Autodesk Inventor part; units mm, degrees
ref_plane "YZ Plane" through (0, 0, 0) normal (1, 0, 0) x (0, 1, 0)
ref_plane "XZ Plane" through (0, 0, 0) normal (0, 1, 0) x (-1, 0, 0)
ref_plane "XY Plane" through (0, 0, 0) normal (0, 0, 1) x (1, 0, 0)
sketch "Sketch1" plane through (0, 0, 0) normal (0, 0, 1) x (1, 0, 0)
  line L0 (-6.55, 3.425) -> (6.55, 3.425)
  line L1 (6.55, 3.425) -> (6.55, -3.425)
  line L2 (6.55, -3.425) -> (-6.55, -3.425)
  line L3 (-6.55, -3.425) -> (-6.55, 3.425)
  point P0 (0, 0)
  dimension "d0" = 13.1
  dimension "d1" = 6.85
  dimension "d2" = 3.425
  dimension "d3" = 6.55
extrude "Extrusion1" add sketch "Sketch1" along normal blind 14.15
sketch "Sketch2" plane through (0, 0, 14.15) normal (0, 0, 1) x (1, 0, 0)
  line L0 (-6, 2.5343) -> (6, 2.5343)
  line L1 (6, 2.5343) -> (6, -2.425)
  line L2 (6, -2.425) -> (-6, -2.425)
  line L3 (-6, -2.425) -> (-6, 2.5343)
  line L4 (-6.55, -3.425) -> (6.55, -3.425)
  line L5 (6.55, 3.425) -> (-6.55, 3.425)
  point P0 (0, 0)
  dimension "d7" = 12
  dimension "d8" = 6
  dimension "d9" = 1
extrude "Extrusion2" cut sketch "Sketch2" against normal blind 10
sketch "Sketch3" plane through (0, 0, 4.15) normal (0, 0, 1) x (1, 0, 0)
  line L0 (-4.7039, 1.4576) -> (5.0017, 1.4576)
  line L1 (5.0017, 1.4576) -> (5.0017, 0.3455)
  line L2 (5.0017, 0.3455) -> (-4.7039, 0.3455)
  line L3 (-4.7039, 0.3455) -> (-4.7039, 1.4576)
  point P0 (0, 0)
extrude "Extrusion3" add sketch "Sketch3" along normal blind 8
sketch "Sketch4" plane through (6.55, -3.425, 0) normal (1, 0, 0) x (0, 0, -1)
  line L0 (-4.85, 2.838) -> (-2.85, 2.838)
  line L1 (-2.85, 2.838) -> (-2.85, -3.2)
  line L2 (-2.85, -3.2) -> (-4.85, -3.2)
  line L3 (-4.85, -3.2) -> (-4.85, 2.838)
  line L4 (-14.15, 0) -> (-14.15, 6.85)
  arc A0 (-4.85, -2.2) -> (-2.85, -2.2) centre (-3.85, -2.2) ccw
  point P0 (0, 3.425)
  dimension "d17" = 2
  dimension "d18" = 9.3
  dimension "d21" = 3.2
extrude "Extrusion4" add sketch "Sketch4" against normal blind 0.5 contours L0 L1 A0 L3
sketch "Sketch5" plane through (-6.55, -3.425, 0) normal (0, -1, 0) x (1, 0, 0)
  line L0 (13.8244, -1.52) -> (1.8735, -1.52) construction
  line L1 (13.8244, 1.1) -> (1.8735, 1.1) construction
  line L2 (13.1, 4.85) -> (12.6, 4.85)
  circle A0 centre (5.55, 1.1) radius 0.4
  circle A1 centre (7.55, 1.1) radius 0.4
  circle A2 centre (3.05, 1.1) radius 0.4
  circle A3 centre (10.05, 1.1) radius 0.4
  point P0 (6.55, 0)
  dimension "d25" = 2.62
  dimension "d26" = 3.75
  dimension "d29" = 2
  dimension "d30" = 1
  dimension "d31" = 2.5
  dimension "d34" = 2.5
  dimension "d35" = 0.8
  dimension "d36" = 0.8
  dimension "d40" = 0.8
  dimension "d42" = 0.8
extrude "Extrusion5" add sketch "Sketch5" along normal blind 3.2
mirror "Mirror1" about plane through (0, 0, 0) normal (1, 0, 0) of "Extrusion4"
properties part number "USBA_CNC"
Source: CAD feature listing. Evaluate the final solid. Frame: model axes, mm. A direction names the side the tool comes from. Coordinates: 2 decimals unless noted, no trailing zeros. Loops run counter-clockwise (first coordinate to the right, second up) from the corner with the lowest first, then second, coordinate; pieces in that order, holes last. Notation, with made-up numbers: M -18,-28 L -9,-28 A13 ccw -9,-24 Z; hole C 87.5,-23 d8. An arc over 180 degrees is marked long. Put each result on its own line as item: value. Start each with the question number.
1) Contact query for flat-ended pins moving along their axis: pin 1 Ø3 at (x, z) = (3, 11.5) entering from -Y (3 decimals); pin 2 Ø1.5 at (x, y) = (-2, 0.5) entering from +Z. Output: stop coordinate, or through.
2) Pull-direction query (Y, two-part tool) for faces 1 (the face through (-4.704, 1, 8)), 2 (the face through (-6.304, -6.625, 3.828)), 3 (the face through (0, 0, 0)); classes: pulls with the +Y half, pulls with the -Y half, needs draft (parallel to the pull), parting line crosses it, or undercut.
3) Reachability of faces 4 (the face through (-6, 0, 9)), 5 (the face through (0, 3.425, 7)), 6 (the face through (6.05, -5, 4)) from +Z, -Z, +X, -X, +Y, -Y: full face, straight path, thin tool, end or side. Return the list, or none.
4) Cut plane C-C on z = 13.75. Return the cut outline in (x, y) (3 decimals), then the cut area to 3 significant figures.
5) Cut plane B-B on z = 5.25. Give the number of separate pieces and of enclosed holes in the cut face, then the cut area to 3 significant figures.
6) Ray query, L1, parallel to Y at x = 4, z = 10.5 (1 decimal); L2, parallel to X at y = 1.25, z = 11; L3, parallel to X at y = 1.5, z = 6. Return the intervals inside material, ascending. Write a range as from..to.
7) Cut plane A-A on y = -4. Return the cut outline in (x, z).
The answers:
1. pin 1: stops at y = -3.425
1. pin 2: stops at z = 12.15
2. face 1: undercut
2. face 2: pulls with the -Y half
2. face 3: needs draft
3. face 4: +Z
3. face 5: +Z, -Z, +X, -X, +Y
3. face 6: +Z, -Z, -Y
4. outline: M -6.55,-3.425 L 6.55,-3.425 L 6.55,3.425 L -6.55,3.425 Z; hole M -6,-2.425 L 6,-2.425 L 6,2.534 L -6,2.534 Z
4. area: 30.2 mm²
5. separate pieces: 2
5. enclosed holes: 1
5. area: 41.0 mm²
6. L1: y = -3.4..-2.4, 0.3..1.5, 2.5..3.4
6. L2: x = -6.55..-6, -4.7..5, 6..6.55
6. L3: x = -6.55..-6, 6..6.55
7. outline: M -6.55,2.85 L -6.05,2.85 L -6.05,4.85 L -6.55,4.85 Z; C -3.5,1.1 d0.8; C -1,1.1 d0.8; C 1,1.1 d0.8; C 3.5,1.1 d0.8; M 6.05,2.85 L 6.55,2.85 L 6.55,4.85 L 6.05,4.85 Z
